```python
from build123d import *

# Parameters (mm, degrees)
SKETCH1_W           = 98
SKETCH1_H           = 98
BOSS_EXTRUDE1_DEPTH = 10
SKETCH8_W           = 98
SKETCH8_H           = 98
SKETCH8_W_2         = 78
SKETCH8_H_2         = 78
CUT_EXTRUDE5_DEPTH  = 5
SKETCH9_W           = 28
SKETCH9_H           = 50
CUT_EXTRUDE6_DEPTH  = 5
SKETCH11_W          = 22.983747508
SKETCH11_H          = 15.1
CUT_EXTRUDE7_DEPTH  = 8
SKETCH12_W          = 3.3
SKETCH12_H          = 15.1
CUT_EXTRUDE8_DEPTH  = 3
CUT_EXTRUDE10_DEPTH = 16
SKETCH14_R          = 1.5
CUT_EXTRUDE11_DEPTH = 10


with BuildPart() as part:
    # Sketch1 → Boss-Extrude1 (new body)
    with BuildSketch(Plane(origin=(0, 0, 0), x_dir=(1, 0, 0), z_dir=(0, 1, 0))):
        Rectangle(SKETCH1_W, SKETCH1_H)
    extrude(amount=BOSS_EXTRUDE1_DEPTH)

    # Sketch8 → Cut-Extrude5 (cut)
    with BuildSketch(Plane(origin=(0, 10, 0), x_dir=(1, 0, 0), z_dir=(0, 1, 0))):
        Rectangle(SKETCH8_W, SKETCH8_H)
        Rectangle(SKETCH8_W_2, SKETCH8_H_2, mode=Mode.SUBTRACT)
    extrude(amount=-CUT_EXTRUDE5_DEPTH, mode=Mode.SUBTRACT)

    # Sketch9 → Cut-Extrude6 (cut)
    with BuildSketch(Plane(origin=(0, 10, 0), x_dir=(1, 0, 0), z_dir=(0, 1, 0))):
        with Locations((-25, -9)):
            Rectangle(SKETCH9_W, SKETCH9_H)
    extrude(amount=-CUT_EXTRUDE6_DEPTH, mode=Mode.SUBTRACT)

    # Sketch11 → Cut-Extrude7 (cut)
    with BuildSketch(Plane(origin=(0, 10, 0), x_dir=(1, 0, 0), z_dir=(0, 1, 0))):
        with Locations((-27.508126246, 27.5)):
            Rectangle(SKETCH11_W, SKETCH11_H)
    extrude(amount=-CUT_EXTRUDE7_DEPTH, mode=Mode.SUBTRACT)

    # Sketch12 → Cut-Extrude8 (cut)
    with BuildSketch(Plane(origin=(0, 5, 0), x_dir=(1, 0, 0), z_dir=(0, 1, 0))):
        with Locations((-40.65, 27.5)):
            Rectangle(SKETCH12_W, SKETCH12_H)
    extrude(amount=-CUT_EXTRUDE8_DEPTH, mode=Mode.SUBTRACT)

    # Sketch13 → Cut-Extrude10 (cut)
    with BuildSketch(Plane(origin=(0, 10, 0), x_dir=(1, 0, 0), z_dir=(0, 1, 0))):
        with BuildLine():
            Line((-4, -18.5), (32, -18.5))
            ThreePointArc((32, -18.5), (33.414213562, -19.085786438), (34, -20.5))
            Line((34, -20.5), (34, -21.5))
            ThreePointArc((34, -21.5), (33.414213562, -22.914213562), (32, -23.5))
            Line((32, -23.5), (-4, -23.5))
            ThreePointArc((-4, -23.5), (-5.414213562, -22.914213562), (-6, -21.5))
            Line((-6, -21.5), (-6, -20.5))
            ThreePointArc((-6, -20.5), (-5.414213562, -19.085786438), (-4, -18.5))
        make_face()
        with BuildLine():
            Line((-4, -34), (32, -34))
            ThreePointArc((32, -34), (33.414213562, -33.414213562), (34, -32))
            Line((34, -32), (34, -31))
            ThreePointArc((34, -31), (33.414213562, -29.585786438), (32, -29))
            Line((32, -29), (-4, -29))
            ThreePointArc((-4, -29), (-5.414213562, -29.585786438), (-6, -31))
            Line((-6, -31), (-6, -32))
            ThreePointArc((-6, -32), (-5.414213562, -33.414213562), (-4, -34))
        make_face()
        with BuildLine():
            Line((-4, -8), (32, -8))
            ThreePointArc((32, -8), (33.414213562, -8.585786438), (34, -10))
            Line((34, -10), (34, -11))
            ThreePointArc((34, -11), (33.414213562, -12.414213562), (32, -13))
            Line((32, -13), (-4, -13))
            ThreePointArc((-4, -13), (-5.414213562, -12.414213562), (-6, -11))
            Line((-6, -11), (-6, -10))
            ThreePointArc((-6, -10), (-5.414213562, -8.585786438), (-4, -8))
        make_face()
        with BuildLine():
            Line((-4, 2.5), (32, 2.5))
            ThreePointArc((32, 2.5), (33.414213562, 1.914213562), (34, 0.5))
            Line((34, 0.5), (34, -0.5))
            ThreePointArc((34, -0.5), (33.414213562, -1.914213562), (32, -2.5))
            Line((32, -2.5), (-4, -2.5))
            ThreePointArc((-4, -2.5), (-5.414213562, -1.914213562), (-6, -0.5))
            Line((-6, -0.5), (-6, 0.5))
            ThreePointArc((-6, 0.5), (-5.414213562, 1.914213562), (-4, 2.5))
        make_face()
        with BuildLine():
            Line((-4, 13), (32, 13))
            ThreePointArc((32, 13), (33.414213562, 12.414213562), (34, 11))
            Line((34, 11), (34, 10))
            ThreePointArc((34, 10), (33.414213562, 8.585786438), (32, 8))
            Line((32, 8), (-4, 8))
            ThreePointArc((-4, 8), (-5.414213562, 8.585786438), (-6, 10))
            Line((-6, 10), (-6, 11))
            ThreePointArc((-6, 11), (-5.414213562, 12.414213562), (-4, 13))
        make_face()
        with BuildLine():
            Line((-4, 23.5), (32, 23.5))
            ThreePointArc((32, 23.5), (33.414213562, 22.914213562), (34, 21.5))
            Line((34, 21.5), (34, 20.5))
            ThreePointArc((34, 20.5), (33.414213562, 19.085786438), (32, 18.5))
            Line((32, 18.5), (-4, 18.5))
            ThreePointArc((-4, 18.5), (-5.414213562, 19.085786438), (-6, 20.5))
            Line((-6, 20.5), (-6, 21.5))
            ThreePointArc((-6, 21.5), (-5.414213562, 22.914213562), (-4, 23.5))
        make_face()
        with BuildLine():
            Line((-4, 34), (32, 34))
            ThreePointArc((32, 34), (33.414213562, 33.414213562), (34, 32))
            Line((34, 32), (34, 31))
            ThreePointArc((34, 31), (33.414213562, 29.585786438), (32, 29))
            Line((32, 29), (-4, 29))
            ThreePointArc((-4, 29), (-5.414213562, 29.585786438), (-6, 31))
            Line((-6, 31), (-6, 32))
            ThreePointArc((-6, 32), (-5.414213562, 33.414213562), (-4, 34))
        make_face()
    extrude(amount=-CUT_EXTRUDE10_DEPTH, mode=Mode.SUBTRACT)

    # Sketch14 → Cut-Extrude11 (cut)
    with BuildSketch(Plane.XZ):
        with Locations(Location((-44, -44, 0), (0, 0, 270))):
            Circle(SKETCH14_R)
        with Locations(Location((-44, 44, 0), (0, 0, 270))):
            Circle(SKETCH14_R)
        with Locations(Location((44, 44, 0), (0, 0, 270))):
            Circle(SKETCH14_R)
        with Locations(Location((44, -44, 0), (0, 0, 270))):
            Circle(SKETCH14_R)
    extrude(amount=-CUT_EXTRUDE11_DEPTH, mode=Mode.SUBTRACT)


solid = part.part
```
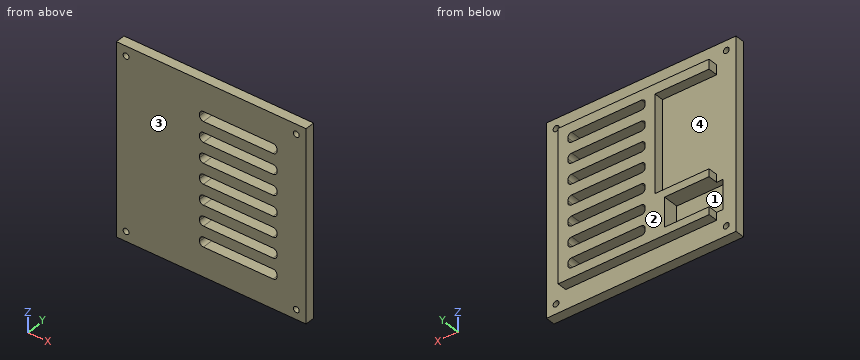
Can you work these out from the model? Positions are in its coordinate system, mm. Face numbers are marked on the shaded views. A direction names the side the tool comes from. Round coordinates to 2 decimals unless told otherwise and drop trailing zeros. Order: outer loops, then holes, each group sorted by start corner. A loop starts at its lowest first (then second) coordinate and runs counter-clockwise, first axis right, second up. Notation, with made-up numbers: (8, 52) -> (58, 52) arc R32 ccw to (58, 84) -> close; hole circle Ø10 at (69.25, 55.5). An arc over 180 degrees is marked (long way). Return JSON: item names as keys, results as strings. Group by question number.
1. If we section it at B-B, the plane x = -44: Write out the boundary of the cut face in (y, z), then the cut area to 3 significant figures.
2. If we section it at C-C, the plane x = 4: Count the separate pieces of the cut face and the enclosed holes in it, then the cut area to 3 significant figures.
3. We'd pull the mould along Z, two halves only. Please class the marked faces 1 and 2: released by +Z, released by -Z, zero draft, split by the parting line, or undercut.
4. If we section it at D-D, the plane z = 15.5: Write out the boundary of the cut face in (x, y), then the cut area to 3 significant figures.
5. Will these pins go through, and if not, where does the flat tip stop? pin 1 (3.5 mm diameter, centred on x = -44, z = -44, fed in from +Y); pin 2 (0.5 mm diameter, centred on y = 7, z = 21, fed in from +X); pin 3 (4 mm diameter, centred on x = 44, z = -44, fed in from -Y); pin 4 (2.5 mm diameter, centred on x = -26.5, y = 6.5, fed in from +Z).
6. Which directions (+Z, -Z, +X, -X, +Y, -Y) give clear straight access to the entire face, cutting with the end or side of a thin tool? Please do the marked faces 3 and 4.
7. If we section it at A-A, the plane z = 44: Write out the boundary of the cut face in (x, y), then the cut area to 3 significant figures.
8. I need wall thicknesses on line 1 (X direction, y = 1.8, z = -44); line 2 (Y direction, x = 41.5, z = -12.5); line 3 (X direction, y = 9.25, z = -18). Which ranges of each line are inside material? Lowest first, please. Write a range as [from, to].
Output values:
{
 "1": {"outline": "(0, -49) -> (5, -49) -> (5, -45.5) -> (0, -45.5) -> close; (0, -42.5) -> (5, -42.5) -> (5, 42.5) -> (0, 42.5) -> close; (0, 45.5) -> (5, 45.5) -> (5, 49) -> (0, 49) -> close", "area": "460 mm²"},
 "2": {"separate pieces": "8", "enclosed holes": "0", "area": "530 mm²"},
 "3": {"face 1": "undercut", "face 2": "zero draft"},
 "4": {"outline": "(-49, 0) -> (49, 0) -> (49, 5) -> (39, 5) -> (39, 10) -> (-11, 10) -> (-11, 5) -> (-49, 5) -> close", "area": "740 mm²"},
 "5": {"pin 1": "y = 5", "pin 2": "x = 39", "pin 3": "y = 0", "pin 4": "z = 39"},
 "6": {"face 3": "+Z, -Z, +X, -X, -Y", "face 4": "+Y"},
 "7": {"outline": "(-49, 0) -> (-45.5, 0) -> (-45.5, 5) -> (-49, 5) -> close; (-42.5, 0) -> (42.5, 0) -> (42.5, 5) -> (-42.5, 5) -> close; (45.5, 0) -> (49, 0) -> (49, 5) -> (45.5, 5) -> close", "area": "460 mm²"},
 "8": {"line 1": "[-49, -45.5], [-42.5, 42.5], [45.5, 49]", "line 2": "[0, 5]", "line 3": "[-39, 39]"}
}
